Could you check a few things on this drawing? It's one solid part, dimensions in mm from its lowest x, y, z. A direction names the side the tool comes from. Round coordinates to 2 decimals unless told otherwise and drop trailing zeros. Order: outer loops, then holes, each group sorted by start corner. A loop starts at its lowest first (then second) coordinate and runs counter-clockwise, first axis right, second up. Notation, with made-up numbers: (-17.75, 32.25) -> (12.25, 32.25) arc R9 cw to (12.25, 49.25) -> close; hole circle Ø1 at (-5, 3.25). An arc over 180 degrees is marked (long way). Use a Markdown table: item, result. Add a question column.
(1) I'm going to push flat-ended pins straight in: P1, Ø7.5, axis at y = 11.5, z = 16.5, coming from the -X side; P2, Ø12.5, axis at x = 8.5, y = 38.5, coming from the +Z side; P3, Ø12.5, axis at y = 12.5, z = 8.5, coming from the +X side. Where does each tip first touch, or does it pass through?
(2) I want a section at D-D, the plane z = 48.5. Please give me the cut outline in (x, y).
(3) On a 3-axis mill with a long thin cutter (end or side, diameter ignored), from which of +Z, -Z, +X, -X, +Y, -Y can I reach the whole of each face in a straight line? I mean the marked faces 1, 2, 3 and 4. Say none if no direction works.
(4) I want a section at C-C, the plane z = 8. Please give me the cut outline in (x, y), then the cut area to 3 significant figures.
(5) I want a section at A-A, the plane y = 33.5. Please give me the cut outline in (x, z).
(6) If I drill on probe 1 along X at (y, z) = (31.5, 41.5); probe 2 along Z at (x, y) = (35.5, 22), over which ranges is the centre line in solid material (lowest first)?
(7) I want a section at B-B, the plane x = 36. Please give me the cut outline in (y, z), then the cut area to 3 significant figures.
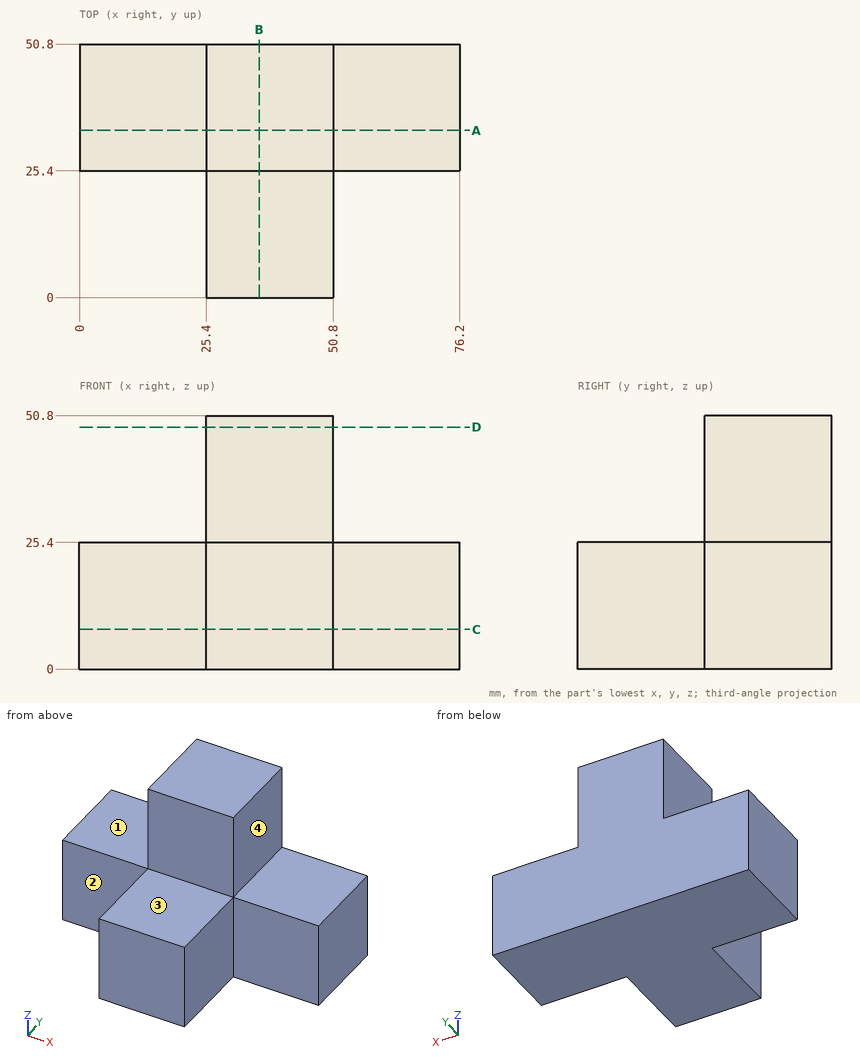
Taken from the geometry:
| question | item | result |
|---|---|---|
| 1 | P1 | stops at x = 25.4 |
| 1 | P2 | stops at z = 25.4 |
| 1 | P3 | stops at x = 50.8 |
| 2 | outline | (25.4, 25.4) -> (50.8, 25.4) -> (50.8, 50.8) -> (25.4, 50.8) -> close |
| 3 | face 1 | +Z, -X, +Y, -Y |
| 3 | face 2 | +Z, -Z, -X, -Y |
| 3 | face 3 | +Z, +X, -X, -Y |
| 3 | face 4 | +Z, +X, +Y, -Y |
| 4 | outline | (0, 25.4) -> (25.4, 25.4) -> (25.4, 0) -> (50.8, 0) -> (50.8, 25.4) -> (76.2, 25.4) -> (76.2, 50.8) -> (0, 50.8) -> close |
| 4 | area | 2,580 mm2 |
| 5 | outline | (0, 0) -> (76.2, 0) -> (76.2, 25.4) -> (50.8, 25.4) -> (50.8, 50.8) -> (25.4, 50.8) -> (25.4, 25.4) -> (0, 25.4) -> close |
| 6 | probe 1 | x = 25.4 to 50.8 |
| 6 | probe 2 | z = 0 to 25.4 |
| 7 | outline | (0, 0) -> (50.8, 0) -> (50.8, 50.8) -> (25.4, 50.8) -> (25.4, 25.4) -> (0, 25.4) -> close |
| 7 | area | 1,940 mm2 |
